from build123d import *

# Parameters (mm, degrees)
F0_W     = 1473.2
F0_H     = 914.4
F1_DEPTH = 1066.8
F2_W     = 1422.4
F2_H     = 863.6
F3_DEPTH = 152.4
F4_W     = 1422.4
F4_H     = 863.6
F5_DEPTH = 863.6
F6_W     = 1422.4
F6_H     = 254
F7_DEPTH = 914.401


with BuildPart() as f1:
    # F0 (on Top) → F1 (new body)
    with BuildSketch(Plane.XY):
        Rectangle(F0_W, F0_H)
    extrude(amount=F1_DEPTH)

    # F2 (on face) → F3 (cut)
    with BuildSketch(Plane.XY.offset(1066.8)):
        with Locations((25.4, -25.4)):
            Rectangle(F2_W, F2_H)
    extrude(amount=-F3_DEPTH, mode=Mode.SUBTRACT)

    # F4 (on face) → F5 (cut)
    with BuildSketch(Plane(origin=(0, 0, 0), x_dir=(1, 0, 0), z_dir=(0, 0, -1))):
        with Locations((25.4, 25.4)):
            Rectangle(F4_W, F4_H)
    extrude(amount=-F5_DEPTH, mode=Mode.SUBTRACT)

    # F6 (on face) → F7 (cut, through all)
    with BuildSketch(Plane.XY.offset(914.4)):
        with Locations((25.4, -330.2)):
            Rectangle(F6_W, F6_H)
    extrude(amount=-F7_DEPTH, mode=Mode.SUBTRACT)


solid = f1.part
The model under review builds one solid part; all positions refer to its coordinate system, in mm. A direction names the side the tool comes from. Round coordinates to 2 decimals unless told otherwise and drop trailing zeros. Order: outer loops, then holes, each group sorted by start corner. A loop starts at its lowest first (then second) coordinate and runs counter-clockwise, first axis right, second up. Notation, with made-up numbers: (40.5, 2.5) -> (87.5, 2.5) arc R19 cw to (87.5, 21.5) -> close; hole circle Ø4 at (-17.75, 49.25). An arc over 180 degrees is marked (long way). Use CSV: the item, a comma, the result in double quotes. Start each with the question number.
(1) Tool access review of faces 1 (the face through (15, -203.2, 889)), 2 (the face through (-10, 457.2, 526)), 3 (the face through (15, 106, 914.4)), 4 (the face through (15, 406.4, 426)): name each direction out of +Z, -Z, +X, -X, +Y, -Y from which nothing blocks a thin tool from reaching the whole face with its end or side.
(2) Consider section B-B on y = -94. Write out the cut boundary in (x, z).
(3) Insertion check: pin 1 (4 mm diameter, centred on y = 357, z = 642.5, fed in from +X); pin 2 (1 mm diameter, centred on x = 394.5, z = 160.5, fed in from -Y); pin 3 (5 mm diameter, centred on x = -151.5, y = -72.5, fed in from -Z). Each pin has a flat end and moves straight along its axis. Give the tip position at first contact, or say it passes through.
(4) Consider section C-C on z = 171.5. Write out the cut boundary in (x, y), and give its area (3 significant figures).
(5) Consider section D-D on z = 881. Write out the cut boundary in (x, y).
(6) Consider section A-A on x = -342.5. Write out the cut boundary in (y, z).
(7) Wall thickness on probe 1 along Z at (x, y) = (374.5, 294.5); probe 2 along Y at (x, z) = (-187, 411.5); probe 3 along X at (y, z) = (170, 95): over which ranges is each line inside the solid? List them lowest first. Write a range as from..to.
Responses:
1,face 1,"+Z, -Z, +X, -Y"
1,face 2,"+Z, -Z, +X, -X, +Y"
1,face 3,"+Z, +X, -Y"
1,face 4,"-Z, +X, -Y"
2,outline,"(-736.6, 0) -> (-685.8, 0) -> (-685.8, 863.6) -> (736.6, 863.6) -> (736.6, 914.4) -> (-685.8, 914.4) -> (-685.8, 1066.8) -> (-736.6, 1066.8) -> close"
3,pin 1,"x = -685.8"
3,pin 2,"y = 406.4"
3,pin 3,"z = 863.6"
4,outline,"(-736.6, -457.2) -> (-685.8, -457.2) -> (-685.8, 406.4) -> (736.6, 406.4) -> (736.6, 457.2) -> (-736.6, 457.2) -> close"
4,area,"119,000 mm²"
5,outline,"(-736.6, -457.2) -> (-685.8, -457.2) -> (-685.8, -203.2) -> (736.6, -203.2) -> (736.6, 457.2) -> (-736.6, 457.2) -> close"
6,outline,"(-203.2, 863.6) -> (406.4, 863.6) -> (406.4, 0) -> (457.2, 0) -> (457.2, 1066.8) -> (406.4, 1066.8) -> (406.4, 914.4) -> (-203.2, 914.4) -> close"
7,probe 1,"863.6..914.4"
7,probe 2,"406.4..457.2"
7,probe 3,"-736.6..-685.8"
